Here's how the part is built. I have some questions about the finished solid (model axes, mm). Face numbers are marked on the shaded views. A direction names the side the tool comes from. Coordinates: 2 decimals unless noted, no trailing zeros. Write each loop counter-clockwise with the first axis right and the second up, starting at its lowest first coordinate (ties: lowest second). Pieces come first, ordered by that corner, then holes.
```python
from build123d import *

# Parameters (mm, degrees)
SKETCH_1_W               = 230
SKETCH_1_H               = 230
EXTRUDE_1_DEPTH          = 3
SKETCH_3_W               = 230
SKETCH_3_H               = 230
EXTRUDE_3_DEPTH          = 100
SKETCH_4_W               = 220
SKETCH_4_H               = 220
CUT_EXTRUDE_1_DEPTH      = 100
SKETCH_6_W               = 20
SKETCH_6_H               = 46
CUT_EXTRUDE_3_DEPTH      = 278.009025124
PATTERN_CIRCULAR_1_COUNT = 2
PATTERN_CIRCULAR_1_ANGLE = 90
SKETCH_11_W              = 224
SKETCH_11_H              = 224
CUT_EXTRUDE_5_DEPTH      = 100
SKETCH_13_W              = 3
SKETCH_13_H              = 56
CUT_EXTRUDE_7_DEPTH      = 278.009025124
SKETCH_14_R              = 2.15
SKETCH_14_W              = 6.4
SKETCH_14_H              = 40
SKETCH_14_W_2            = 40
SKETCH_14_H_2            = 6.4
CUT_EXTRUDE_8_DEPTH      = 191.91883092
PATTERN_CIRCULAR_2_COUNT = 2
PATTERN_CIRCULAR_2_ANGLE = 90


with BuildPart() as part:
    # 스케치1 → 보스-돌출1 (new body)
    with BuildSketch(Plane.XY):
        Rectangle(SKETCH_1_W, SKETCH_1_H)
    extrude(amount=EXTRUDE_1_DEPTH)

    # 스케치3 → 보스-돌출3 (add)
    with BuildSketch(Plane.XY.offset(3)):
        Rectangle(SKETCH_3_W, SKETCH_3_H)
    extrude(amount=EXTRUDE_3_DEPTH)

    # 스케치4 → 컷-돌출1 (cut)
    with BuildSketch(Plane.XY.offset(103)):
        Rectangle(SKETCH_4_W, SKETCH_4_H)
    extrude(amount=-CUT_EXTRUDE_1_DEPTH, mode=Mode.SUBTRACT)

    # 스케치6 → 컷-돌출3 (cut, through all)
    with BuildSketch(Plane.ZY.offset(115)):
        with Locations((73, 0)):
            Rectangle(SKETCH_6_W, SKETCH_6_H)
    cut_extrude_3 = extrude(amount=-CUT_EXTRUDE_3_DEPTH, mode=Mode.SUBTRACT)

    # 원형 패턴1: 컷-돌출3 ×2 about axis
    pattern_circular_1_axis = Axis((0, 0, 0), (0, 0, 1))
    for i in range(1, PATTERN_CIRCULAR_1_COUNT):
        add(cut_extrude_3.rotate(pattern_circular_1_axis, i * PATTERN_CIRCULAR_1_ANGLE / (PATTERN_CIRCULAR_1_COUNT - 1)), mode=Mode.SUBTRACT)

    # 스케치11 → 컷-돌출5 (cut)
    with BuildSketch(Plane.XY.offset(103)):
        Rectangle(SKETCH_11_W, SKETCH_11_H)
    extrude(amount=-CUT_EXTRUDE_5_DEPTH, mode=Mode.SUBTRACT)

    # 스케치13 → 컷-돌출7 (cut, through all)
    with BuildSketch(Plane.ZY.offset(115)):
        with Locations((101.5, 0)):
            Rectangle(SKETCH_13_W, SKETCH_13_H)
    cut_extrude_7 = extrude(amount=-CUT_EXTRUDE_7_DEPTH, mode=Mode.SUBTRACT)

    # 스케치14 → 컷-돌출8 (cut, through all)
    with BuildSketch(Plane.XY.offset(3)):
        with Locations((-106, -34)):
            Circle(SKETCH_14_R)
        with Locations((-106, 34)):
            Circle(SKETCH_14_R)
        with Locations((-34, 106)):
            Circle(SKETCH_14_R)
        with Locations((34, 106)):
            Circle(SKETCH_14_R)
        with Locations((106, 34)):
            Circle(SKETCH_14_R)
        with Locations((106, -34)):
            Circle(SKETCH_14_R)
        with Locations((34, -106)):
            Circle(SKETCH_14_R)
        with Locations((-34, -106)):
            Circle(SKETCH_14_R)
        with Locations((-103, 0)):
            Rectangle(SKETCH_14_W, SKETCH_14_H)
        with Locations((0, 103)):
            Rectangle(SKETCH_14_W_2, SKETCH_14_H_2)
        with Locations((103, 0)):
            Rectangle(SKETCH_14_W, SKETCH_14_H)
        with Locations((0, -103)):
            Rectangle(SKETCH_14_W_2, SKETCH_14_H_2)
    extrude(amount=-CUT_EXTRUDE_8_DEPTH, mode=Mode.SUBTRACT)

    # 원형 패턴2: 컷-돌출7 ×2 about axis
    pattern_circular_2_axis = Axis((0, 0, -18.105724747), (0, 0, 1))
    for i in range(1, PATTERN_CIRCULAR_2_COUNT):
        add(cut_extrude_7.rotate(pattern_circular_2_axis, i * PATTERN_CIRCULAR_2_ANGLE / (PATTERN_CIRCULAR_2_COUNT - 1)), mode=Mode.SUBTRACT)


solid = part.part
```
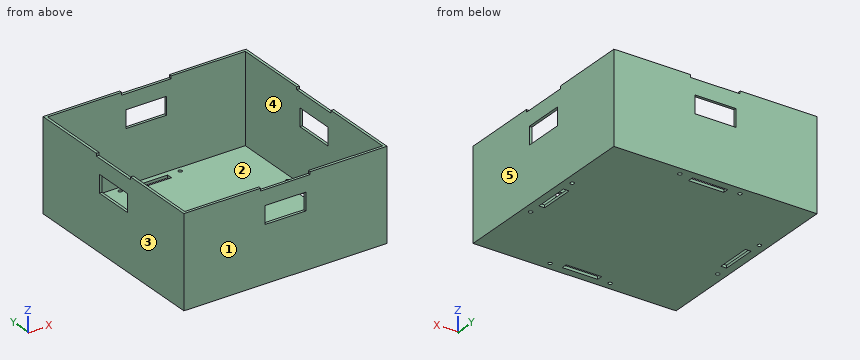
1) I need wall thicknesses on probe 1 along Y at (x, z) = (-34, 1.3); probe 2 along Y at (x, z) = (106, 2.3); probe 3 along Y at (x, z) = (-63, 42.5). Which ranges of each line are inside material? Lowest first, please.
Values follow:
probe 1: y = -115 to -108.15, -103.85 to 103.85, 108.15 to 115
probe 2: y = -115 to -36.15, -31.85 to -20, 20 to 31.85, 36.15 to 115
probe 3: y = -115 to -112, 112 to 115
2) Imagine slicing it at C-C on x = -46.5. Please give me the cut outline in (y, z).
Values follow:
outline: (-115, 0) - (115, 0) - (115, 103) - (112, 103) - (112, 3) - (-112, 3) - (-112, 103) - (-115, 103) - close
3) Imagine slicing it at B-B on z = 32. Please give me the cut outline in (x, y).
Values follow:
outline: (-115, -115) - (115, -115) - (115, 115) - (-115, 115) - close; hole (-112, -112) - (112, -112) - (112, 112) - (-112, 112) - close
4) We'd pull the mould along X, two halves only. Please class the marked faces 1, 2 and 3: pulls with the +X half, pulls with the -X half, needs draft (parallel to the pull), parting line crosses it, or undercut.
Values follow:
face 1: needs draft
face 2: undercut
face 3: pulls with the -X half
5) On a 3-axis mill with a long thin cutter (end or side, diameter ignored), from which of +Z, -Z, +X, -X, +Y, -Y can I reach the whole of each face in a straight line? I mean the marked faces 4 and 5. Say none if no direction works.
Values follow:
face 4: +Z
face 5: +Z, -Z, +X, +Y, -Y
6) Imagine slicing it at A-A on z = 77. Please give me the cut outline in (x, y), then the cut area to 3 significant figures.
Values follow:
outline: (-115, -115) - (-23, -115) - (-23, -112) - (-112, -112) - (-112, -23) - (-115, -23) - close; (-115, 23) - (-112, 23) - (-112, 112) - (-23, 112) - (-23, 115) - (-115, 115) - close; (23, -115) - (115, -115) - (115, -23) - (112, -23) - (112, -112) - (23, -112) - close; (23, 112) - (112, 112) - (112, 23) - (115, 23) - (115, 115) - (23, 115) - close
area: 2,170 mm2
7) Will these pins go through, and if not, where does the flat tip stop? pin 1 (6 mm diameter, centred on x = -34.5, y = -14, fed in from +Z); pin 2 (2.5 mm diameter, centred on x = 113, y = 10.5, fed in from +Z).
Values follow:
pin 1: stops at z = 3
pin 2: stops at z = 100
